Build history of the part. All positions in model axes, mm. Face numbers are marked on the shaded views. A direction names the side the tool comes from. Give positions to 0.01 mm unless a question says otherwise; leave off trailing zeros. Loops run counter-clockwise (first coordinate to the right, second up) from the corner with the lowest first, then second, coordinate; pieces in that order, holes last.
1) 3-axis set-ups, long thin cutter, end or side, ignore diameter. For the marked faces 1 and 2: which of +Z, -Z, +X, -X, +Y, -Y reach the whole face in a straight line?
2) Wall check: line 1 (X direction, y = 3, z = -2.8); line 2 (Z direction, x = -7.5, y = 1.1); line 3 (Y direction, x = -2.5, z = -7.5). Give the ranges that are in metal, low to high.
3) Two-plate mould, pull along Z, no slides. Class the marked faces 3, 4 and 5: +Z half, -Z half, draft (parallel to the pull), parting line (faces both ways), or undercut.
4) Flat gauge pins, fed straight in: P1, Ø3, axis at x = -5, z = -11.5, coming from the -Y side; P2, Ø0.5, axis at x = -6.5, y = 0.5, coming from the -Z side; P3, Ø1.9, axis at x = -7.5, z = -25, coming from the -Y side. Where does each tip first touch, or does it go through?
5) Band-saw the part on A-A on x = -7.5. List the corners of the cut face in (y, z).
6) Band-saw the part on B-B on y = 1.45. List the corners of the cut face in (x, z).
7) Band-saw the part on D-D on x = -14.5. List the corners of the cut face in (y, z), then the cut area to 3 significant figures.
8) Band-saw the part on C-C on z = -2.8. List the corners of the cut face in (x, y), then the cut area to 3 significant figures.
Autodesk Inventor part; units mm, degrees
ref_plane "YZ Plane" through (0, 0, 0) normal (1, 0, 0) x (0, 1, 0)
ref_plane "XZ Plane" through (0, 0, 0) normal (0, 1, 0) x (-1, 0, 0)
ref_plane "XY Plane" through (0, 0, 0) normal (0, 0, 1) x (1, 0, 0)
sketch "Эскиз1" plane through (0, 0, 0) normal (0, 1, 0) x (-1, 0, 0)
  line L0 (17.5, -26.75) -> (-2.5, -26.75)
  line L1 (17.5, -26.75) -> (17.5, -2.5)
  line L2 (15, 0) -> (17.5, -2.5)
  line L3 (0, 0) -> (15, 0)
  line L4 (-2.5, -2.5) -> (0, 0)
  line L5 (-2.5, -26.75) -> (-2.5, -2.5)
  circle A0 centre (7.5, -2.8) radius 1.6
  circle A1 centre (7.5, -25) radius 1.6
  point P0 (7.5, -40)
extrude "Выдавливание1" add sketch "Эскиз1" along normal blind 5
sketch "Эскиз2" plane through (0, 0, 0) normal (0, -1, 0) x (1, 0, 0)
  line L0 (2.5, -2.5) -> (2.5, -26.75)
  line L1 (-17.5, -26.75) -> (-17.5, -2.5)
  line L2 (2.5, -7.2576) -> (-17.5, -7.2576)
  line L3 (-17.5, -7.2576) -> (-17.5, -13.2576)
  line L4 (-17.5, -13.2576) -> (2.5, -13.2576)
  line L5 (2.5, -13.2576) -> (2.5, -7.2576)
  point P0 (0, 0)
  dimension "d2" = 6
extrude "Выдавливание2" cut sketch "Эскиз2" against normal blind 1
move faces "Перенос1" translate (0, 0, -3) faces at (-4.1667, 1.6667, -26.75)
chamfer "Фаска1" distance 2 angle 45 1 edges at (-7.5, 0, -29.75)
properties part number "КВ33.044.202 - Прижим ремня" material "Пластик АБС"
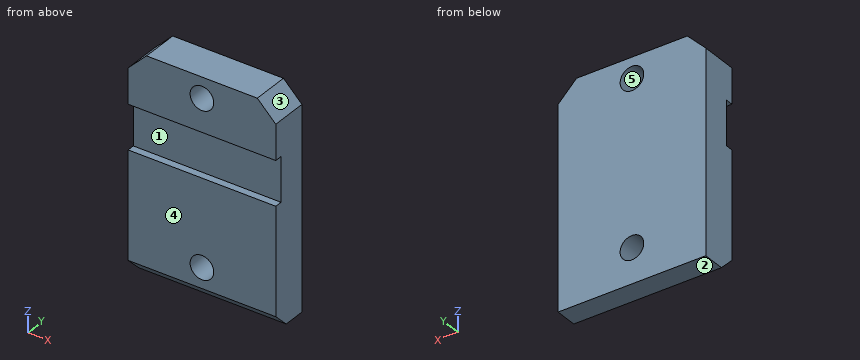
Findings below:
1. face 1: +X, -X, -Y
1. face 2: -Z, +X, -X, +Y, -Y
2. line 1: x = -17.5 to -9.1, -5.9 to 2.5
2. line 2: z = -28.85 to -26.6, -23.4 to -4.4, -1.2 to 0
2. line 3: y = 1 to 5
3. face 3: +Z half
3. face 4: draft
3. face 5: undercut
4. P1: stops at y = 1
4. P2: stops at z = -28.5
4. P3: passes through
5. outline: (0, -27.75) - (2, -29.75) - (5, -29.75) - (5, -26.6) - (0, -26.6) - close; (0, -23.4) - (5, -23.4) - (5, -4.4) - (0, -4.4) - (0, -7.26) - (1, -7.26) - (1, -13.26) - (0, -13.26) - close; (0, -1.2) - (5, -1.2) - (5, 0) - (0, 0) - close
6. outline: (-17.5, -29.2) - (2.5, -29.2) - (2.5, -2.5) - (0, 0) - (-15, 0) - (-17.5, -2.5) - close; hole circle Ø3.2 at (-7.5, -25); hole circle Ø3.2 at (-7.5, -2.8)
7. outline: (0, -27.75) - (2, -29.75) - (5, -29.75) - (5, 0) - (0, 0) - (0, -7.26) - (1, -7.26) - (1, -13.26) - (0, -13.26) - close
7. area: 141 mm2
8. outline: (-17.5, 0) - (-9.1, 0) - (-9.1, 5) - (-17.5, 5) - close; (-5.9, 0) - (2.5, 0) - (2.5, 5) - (-5.9, 5) - close
8. area: 84.0 mm2
